```python
from build123d import *

# Parameters (mm, degrees)
SKETCH1_W           = 200
SKETCH1_H           = 200
BOSS_EXTRUDE1_DEPTH = 10
SKETCH2_R           = 3.5
CUT_EXTRUDE1_DEPTH  = 11
SKETCH3_R           = 6
CUT_EXTRUDE2_DEPTH  = 11


with BuildPart() as part:
    # Sketch1 → Boss-Extrude1 (new body)
    with BuildSketch(Plane(origin=(0, 0, 0), x_dir=(1, 0, 0), z_dir=(0, 1, 0))):
        Rectangle(SKETCH1_W, SKETCH1_H)
    extrude(amount=BOSS_EXTRUDE1_DEPTH)

    # Sketch2 → Cut-Extrude1 (cut, through all)
    with BuildSketch(Plane(origin=(0, 10, 0), x_dir=(1, 0, 0), z_dir=(0, 1, 0))):
        with Locations((45, 75)):
            Circle(SKETCH2_R)
    extrude(amount=-CUT_EXTRUDE1_DEPTH, mode=Mode.SUBTRACT)

    # Sketch3 → Cut-Extrude2 (cut, through all)
    with BuildSketch(Plane(origin=(0, 10, 0), x_dir=(1, 0, 0), z_dir=(0, 1, 0))):
        with Locations((-45, 75)):
            Circle(SKETCH3_R)
    extrude(amount=-CUT_EXTRUDE2_DEPTH, mode=Mode.SUBTRACT)


solid = part.part
```
Design review of the part built by this model. Coordinates are the model's own, in mm. Give positions to 0.01 mm unless a question says otherwise; leave off trailing zeros. Write each loop counter-clockwise with the first axis right and the second up, starting at its lowest first coordinate (ties: lowest second). Pieces come first, ordered by that corner, then holes. Notation, with made-up numbers: (45, -36) -> (84, -36) arc R16 ccw to (84, -15) -> close; hole circle Ø11 at (17.25, 40.5). An arc over 180 degrees is marked (long way). Answer in a Markdown table with one row per item.
(1) Consider section C-C (x = -45). State the section outline as (y, z) points.
Results:
| item | result |
|---|---|
| outline | (0, -100) -> (10, -100) -> (10, -81) -> (0, -81) -> close; (0, -69) -> (10, -69) -> (10, 100) -> (0, 100) -> close |
(2) Consider section A-A (x = 45). State the section outline as (y, z) points, then the cut area to 3 significant figures.
Results:
| item | result |
|---|---|
| outline | (0, -100) -> (10, -100) -> (10, -78.5) -> (0, -78.5) -> close; (0, -71.5) -> (10, -71.5) -> (10, 100) -> (0, 100) -> close |
| area | 1,930 mm2 |
(3) To check wall thickness, follow probe 1 along X at (y, z) = (8, -75); probe 2 along Z at (x, y) = (45, 4.25); probe 3 along Z at (x, y) = (-45, 3.75). State the ranges of each line that lie inside material, in increasing order.
Results:
| item | result |
|---|---|
| probe 1 | -100 to -51, -39 to 41.5, 48.5 to 100 |
| probe 2 | -100 to -78.5, -71.5 to 100 |
| probe 3 | -100 to -81, -69 to 100 |
(4) Mouldability with a two-part tool opening along Z and no side actions: class faces 1 (the flat face through (-1, 5, -100)), 2 (the cylindrical face through (42.2, 5.1, -72.9)), 3 (the flat face through (-1, 0, -1)) as +Z half, -Z half, draft (parallel to the pull), parting line (faces both ways), or undercut.
Results:
| item | result |
|---|---|
| face 1 | -Z half |
| face 2 | undercut |
| face 3 | draft |
(5) Consider section B-B (z = -75). State the section outline as (x, y) points.
Results:
| item | result |
|---|---|
| outline | (-100, 0) -> (-51, 0) -> (-51, 10) -> (-100, 10) -> close; (-39, 0) -> (41.5, 0) -> (41.5, 10) -> (-39, 10) -> close; (48.5, 0) -> (100, 0) -> (100, 10) -> (48.5, 10) -> close |
